```python
from build123d import *

# Parameters (mm, degrees)
SKETCH1_W           = 40
SKETCH1_H           = 70
SKETCH1_R           = 7.5
BOSS_EXTRUDE1_DEPTH = 40
CUT_EXTRUDE1_DEPTH  = 20
SKETCH3_W           = 40
SKETCH3_H           = 40
CUT_EXTRUDE2_DEPTH  = 20
FILLET1_R           = 15


with BuildPart() as part:
    # Sketch1 → Boss-Extrude1 (new body)
    with BuildSketch(Plane.XY):
        with Locations((0, 15)):
            Rectangle(SKETCH1_W, SKETCH1_H)
        Circle(SKETCH1_R, mode=Mode.SUBTRACT)
    extrude(amount=BOSS_EXTRUDE1_DEPTH)

    # Sketch2 → Cut-Extrude1 (cut)
    with BuildSketch(Plane(origin=(0, 50, 0), x_dir=(1, 0, 0), z_dir=(0, 1, 0))):
        with BuildLine():
            ThreePointArc((7.5, -20), (2.870125743, -13.070903506), (-5.303300859, -14.696699141))
            Line((-5.303300859, -14.696699141), (5.303300859, -25.303300859))
            ThreePointArc((5.303300859, -25.303300859), (6.929096494, -22.870125743), (7.5, -20))
        make_face()
        with BuildLine():
            Line((5.303300859, -25.303300859), (-5.303300859, -14.696699141))
            ThreePointArc((-5.303300859, -14.696699141), (-5.303300859, -25.303300859), (5.303300859, -25.303300859))
        make_face()
    extrude(amount=-CUT_EXTRUDE1_DEPTH, mode=Mode.SUBTRACT)

    # Sketch3 → Cut-Extrude2 (cut)
    with BuildSketch(Plane.XY.offset(40)):
        Rectangle(SKETCH3_W, SKETCH3_H)
    extrude(amount=-CUT_EXTRUDE2_DEPTH, mode=Mode.SUBTRACT)

    # Fillet1
    fillet1_edges = [part.edges().sort_by_distance(p)[0] for p in [
        (20, -20, 10),
        (-20, -20, 10),
        (-20, 20, 30),
        (20, 20, 30),
    ]]
    fillet(fillet1_edges, radius=FILLET1_R)


solid = part.part
```
Design review of the part built by this model. Coordinates are the model's own, in mm. A direction names the side the tool comes from. Give positions to 0.01 mm unless a question says otherwise; leave off trailing zeros. Order: outer loops, then holes, each group sorted by start corner. A loop starts at its lowest first (then second) coordinate and runs counter-clockwise, first axis right, second up. Notation, with made-up numbers: (73, 11.5) -> (80, 11.5) arc R19 cw to (80, 28.5) -> close; hole circle Ø9 at (0, 47). An arc over 180 degrees is marked (long way). Write each question's results on one line, items separated by ' | '. Start each with the question number.
Q1. Add section A-A on x = 0. Give the boundary of the cut face in (y, z).
Q2. Add section B-B on z = 4. Give the boundary of the cut face in (x, y), and give its area (3 significant figures).
Q3. Mouldability with a two-part tool opening along Z and no side actions: class faces 1 (the flat face through (0, 30, 20)), 2 (the flat face through (0, 20, 30)), 3 (the flat face through (0, 8, 20)) as +Z half, -Z half, draft (parallel to the pull), parting line (faces both ways), or undercut.
Q4. Machinability: for faces 4 (the cylindrical face through (15.49, 24.28, 29.86)), 5 (the cylindrical face through (-15.72, 24.51, 29.86)), 6 (the flat face through (-20, 28, 15)), which of the approach directions +Z, -Z, +X, -X, +Y, -Y give a long, thin tool a straight path to every point of the face, cutting with its end or side? Answer none if there is none.
Q5. Add section C-C on y = 0. Give the boundary of the cut face in (x, z).
Q6. For pin 1 (7.5 mm diameter, centred on x = -0.5, z = 21, fed in from +Y); pin 2 (4 mm diameter, centred on y = 30, z = 26, fed in from +X); pin 3 (17 mm diameter, centred on x = 0, y = 0, fed in from +Z), all flat-tipped, find the tip position at first contact; note any pin that passes through.
Q7. Wall thickness on L1, parallel to X at y = 0, z = 6.5; L2, parallel to Y at x = 0, z = 9.75; L3, parallel to Y at x = 0, z = 13.25: over which ranges is each line inside the solid? List them lowest first. Write a range as from..to.
Q8. Add section D-D on z = 32. Give the boundary of the cut face in (x, y), and give its area (3 significant figures).
Found:
1) outline: (-20, 0) -> (-7.5, 0) -> (-7.5, 20) -> (-20, 20) -> close; (7.5, 0) -> (50, 0) -> (50, 12.5) -> (30, 12.5) -> (30, 27.5) -> (50, 27.5) -> (50, 40) -> (20, 40) -> (20, 20) -> (7.5, 20) -> close
2) outline: (-20, -5) arc R15 ccw to (-5, -20) -> (5, -20) arc R15 ccw to (20, -5) -> (20, 50) -> (-20, 50) -> close; hole circle Ø15 at (0, 0) | area: 2,530 mm2
3) face 1: undercut | face 2: draft | face 3: +Z half
4) face 4: +Z, +X, -Y | face 5: +Z, -X, -Y | face 6: +Z, -Z, -X, +Y, -Y
5) outline: (-20, 0) -> (-7.5, 0) -> (-7.5, 20) -> (-20, 20) -> close; (7.5, 0) -> (20, 0) -> (20, 20) -> (7.5, 20) -> close
6) pin 1: stops at y = 30 | pin 2: stops at x = 19.7 | pin 3: stops at z = 20
7) L1: x = -20..-7.5, 7.5..20 | L2: y = -20..-7.5, 7.5..50 | L3: y = -20..-7.5, 7.5..30
8) outline: (-20, 35) arc R15 ccw to (-5, 20) -> (5, 20) arc R15 ccw to (20, 35) -> (20, 50) -> (-20, 50) -> close | area: 1,100 mm2
